For this review, take the finished solid that the model builds, in its own axes (mm). Face numbers are marked on the shaded views. Coordinates: 2 decimals unless noted, no trailing zeros. Order: outer loops, then holes, each group sorted by start corner. A loop starts at its lowest first (then second) coordinate and runs counter-clockwise, first axis right, second up. Notation, with made-up numbers: M 48,11.25 L 74,11.25 A28 cw 74,50.25 Z; hole C -17,26.5 d10. An arc over 180 degrees is marked long. Use CSV: the item, a comma, the result in double quotes.
```python
from build123d import *

# Parameters (mm, degrees)
F1_DEPTH = 3.5
F2_DEPTH = 2
F3_DEPTH = 1.5


with BuildPart() as f1:
    # F0 (on Top) → F1 (new body, symmetric)
    with BuildSketch(Plane.XY):
        Polygon((15.5, 13.61), (15.5, -8.5), (18.5, -8.5), (18.5, 20.237967), (-24.5, 20.237967), (-24.5, -8.5), (-15.5, -8.5), (-15.5, 13.61), align=None)
    extrude(amount=F1_DEPTH, both=True)

    # F0 (on Top) → F2 (join)
    with BuildSketch(Plane.XY):
        Polygon((8.207107, 9), (14.5, 2.707107), (14.5, -8.5), (15.5, -8.5), (15.5, 13.61), (-15.5, 13.61), (-15.5, -8.5), (-14.5, -8.5), (-14.5, 2.707107), (-8.207107, 9), align=None)
    extrude(amount=-F2_DEPTH)

    # F1_face (on face) → F3 (cut)
    with BuildSketch(Plane(origin=(-6.736408, 9.996449, -3.5), x_dir=(1, 0, 0), z_dir=(0, 0, -1))):
        Polygon((22.236408, 18.496449), (22.236408, -3.613551), (-8.763592, -3.613551), (-8.763592, 18.496449), (-17.763592, 18.496449), (-17.763592, -10.241518), (25.236408, -10.241518), (25.236408, 18.496449), align=None)
    extrude(amount=-F3_DEPTH, mode=Mode.SUBTRACT)


solid = f1.part
```
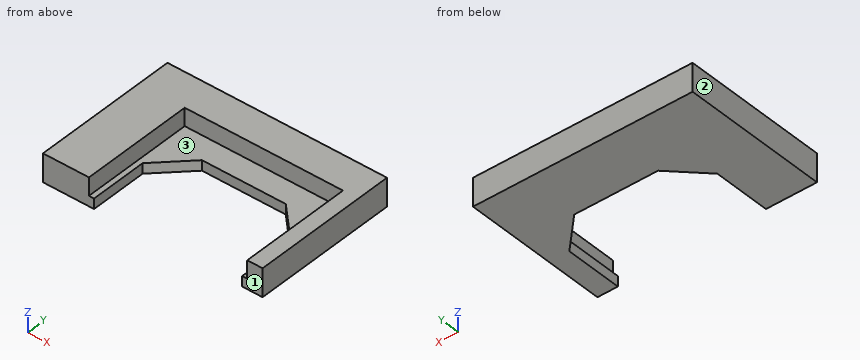
Item 1: Add section C-C on x = 4.5. State the section outline as (y, z) points, and give its area (3 significant figures).
Solutions:
outline,"M 9,-2 L 20.24,-2 L 20.24,3.5 L 13.61,3.5 L 13.61,0 L 9,0 Z"
area,"45.7 mm^2"
Item 2: Draft analysis for pull direction X (two halves, no side actions). For the marked faces 1, 2 and 3, state which applies: released by +X, released by -X, zero draft, split by the parting line, or undercut.
Solutions:
face 1,"zero draft"
face 2,"released by -X"
face 3,"undercut"
Item 3: Add section D-D on y = -4.5. State the section outline as (x, z) points, and give its area (3 significant figures).
Solutions:
outline,"M -24.5,-2 L -14.5,-2 L -14.5,0 L -15.5,0 L -15.5,3.5 L -24.5,3.5 Z; M 14.5,-2 L 18.5,-2 L 18.5,3.5 L 15.5,3.5 L 15.5,0 L 14.5,0 Z"
area,"70.0 mm^2"
Item 4: Add section B-B on z = -0.75. State the section outline as (x, y) points, and give its area (3 significant figures).
Solutions:
outline,"M -24.5,-8.5 L -14.5,-8.5 L -14.5,2.71 L -8.21,9 L 8.21,9 L 14.5,2.71 L 14.5,-8.5 L 18.5,-8.5 L 18.5,20.24 L -24.5,20.24 Z"
area,"768 mm^2"
Item 5: To check wall thickness, follow line 1 along X through (y, z) = (-4, -0.1); line 2 along X through (y, z) = (-2.5, 2.3); line 3 along Y through (x, z) = (-12, 3.1). State the ranges of each line that lie inside material, in increasing order. Write a range as [from, to].
Solutions:
line 1,"[-24.5, -14.5], [14.5, 18.5]"
line 2,"[-24.5, -15.5], [15.5, 18.5]"
line 3,"[13.61, 20.24]"
Item 6: Add section A-A on y = 5.5. State the section outline as (x, z) points, and give its area (3 significant figures).
Solutions:
outline,"M -24.5,-2 L -11.71,-2 L -11.71,0 L -15.5,0 L -15.5,3.5 L -24.5,3.5 Z; M 11.71,-2 L 18.5,-2 L 18.5,3.5 L 15.5,3.5 L 15.5,0 L 11.71,0 Z"
area,"81.2 mm^2"
Item 7: Clearance check with flat-ended pins moving along their axes: pin 1 Ø1 at (x, z) = (-3, 1) entering from -Y; pin 2 Ø2 at (x, z) = (3, -1) entering from -Y; pin 3 Ø10 at (x, y) = (-6.5, 6) entering from +Z. State where each tip first meets the part, or that it passes through.
Solutions:
pin 1,"y = 13.61"
pin 2,"y = 9"
pin 3,"z = 0"
